```python
from build123d import *

# Parameters (mm, degrees)
SKETCH1_R           = 3.175
BOSS_EXTRUDE1_DEPTH = 6.35


with BuildPart() as part:
    # Sketch1 → Boss-Extrude1 (new body)
    with BuildSketch(Plane.XY):
        Polygon((-63.5, 12.7), (-63.5, 6.35), (-69.85, 6.35), (-69.85, -6.35), (-63.5, -6.35), (-63.5, -12.7), (-57.15, -12.7), (-57.15, -6.35), (-50.8, -6.35), (-50.8, -12.7), (-44.45, -12.7), (-44.45, -6.35), (-38.1, -6.35), (-38.1, -12.7), (-31.75, -12.7), (-31.75, -6.35), (-25.4, -6.35), (-25.4, -12.7), (-19.05, -12.7), (-19.05, -6.35), (-12.7, -6.35), (-12.7, -12.7), (-6.35, -12.7), (-6.35, -6.35), (0, -6.35), (6.35, -6.35), (6.35, -12.7), (12.7, -12.7), (12.7, -6.35), (19.05, -6.35), (19.05, -12.7), (25.4, -12.7), (25.4, -6.35), (31.75, -6.35), (31.75, -12.7), (38.1, -12.7), (38.1, -6.35), (44.45, -6.35), (44.45, -12.7), (50.8, -12.7), (50.8, -6.35), (57.15, -6.35), (57.15, -12.7), (63.5, -12.7), (63.5, -6.35), (69.85, -6.35), (69.85, 6.35), (63.5, 6.35), (63.5, 12.7), (57.15, 12.7), (57.15, 6.35), (50.8, 6.35), (50.8, 12.7), (44.45, 12.7), (44.45, 6.35), (38.1, 6.35), (38.1, 12.7), (31.75, 12.7), (31.75, 6.35), (25.4, 6.35), (25.4, 12.7), (19.05, 12.7), (19.05, 6.35), (12.7, 6.35), (12.7, 12.7), (6.35, 12.7), (6.35, 6.35), (0, 6.35), (-6.35, 6.35), (-6.35, 12.7), (-12.7, 12.7), (-12.7, 6.35), (-19.05, 6.35), (-19.05, 12.7), (-25.4, 12.7), (-25.4, 6.35), (-31.75, 6.35), (-31.75, 12.7), (-38.1, 12.7), (-38.1, 6.35), (-44.45, 6.35), (-44.45, 12.7), (-50.8, 12.7), (-50.8, 6.35), (-57.15, 6.35), (-57.15, 12.7), align=None)
        with Locations((-50.8, 0)):
            Circle(SKETCH1_R, mode=Mode.SUBTRACT)
        with Locations((50.8, 0)):
            Circle(SKETCH1_R, mode=Mode.SUBTRACT)
    extrude(amount=BOSS_EXTRUDE1_DEPTH)


solid = part.part
```
Geometry check sheet. Reference: the model listing, model coordinates, mm. A direction names the side the tool comes from. Round coordinates to 2 decimals unless told otherwise and drop trailing zeros. Order: outer loops, then holes, each group sorted by start corner. A loop starts at its lowest first (then second) coordinate and runs counter-clockwise, first axis right, second up. Notation, with made-up numbers: (-2, 2.5) - (4, 2.5) arc R20 ccw to (4, 15.5) - close; hole circle Ø7 at (-17, 75.25). An arc over 180 degrees is marked (long way). Use a Markdown table: item, result. Add a question column.
(1) Material ranges on line 1 along X through (y, z) = (0.25, 2.25); line 2 along X through (y, z) = (2.25, 3.75); line 3 along Y through (x, z) = (2.5, 4.25), recorded low to high. Write a range as [from, to].
(2) Depth check by flat-ended pin: pin 1 (2 mm diameter, centred on x = 14.5, z = 4, fed in from +Y); pin 2 (8 mm diameter, centred on x = 39, y = -7.5, fed in from -Z); pin 3 (1.9 mm diameter, centred on y = -8.5, z = 3.5, fed in from +X); pin 4 (3 mm diameter, centred on y = 9, z = 4.5, fed in from -X). Enter the tip coordinate at first touch or a pass-through.
(3) Tool access check on faces 1 (the flat face through (41, -6.35, 3)), 2 (the flat face through (-6.35, 9, 3)), 3 (the flat face through (-67, -6.35, 3)). Record the directions out of +Z, -Z, +X, -X, +Y, -Y that give a thin tool (end or side, any length) a straight path to the whole face; none if there is none.
(4) Sectioned sample at B-B, the plane x = -49.5. Enter the section's corners in (y, z), and give its area (3 significant figures).
(5) Sectioned sample at C-C, the plane z = 2. Count the separate pieces of the cut face and the enclosed holes in it, and give its area (3 significant figures).
(6) Sectioned sample at A-A, the plane y = 0. Enter the section's corners in (x, z) (3 decimals).
(7) Release check for a two-part mould opening along X. For faces 4 (the flat face through (57.15, 10, 3)), 5 (the flat face through (69.85, 0, 3)), 6 (the flat face through (48, -12.7, 3)) record: pulls with the +X half, pulls with the -X half, needs draft (parallel to the pull), parting line crosses it, or undercut.
Answers below:
| question | item | result |
|---|---|---|
| 1 | line 1 | [-69.85, -53.97], [-47.63, 47.63], [53.97, 69.85] |
| 1 | line 2 | [-69.85, -53.04], [-48.56, 48.56], [53.04, 69.85] |
| 1 | line 3 | [-6.35, 6.35] |
| 2 | pin 1 | y = 6.35 |
| 2 | pin 2 | z = 0 |
| 2 | pin 3 | x = 63.5 |
| 2 | pin 4 | x = -63.5 |
| 3 | face 1 | +Z, -Z, -Y |
| 3 | face 2 | +Z, -Z, +Y |
| 3 | face 3 | +Z, -Z, -X, -Y |
| 4 | outline | (-12.7, 0) - (-2.9, 0) - (-2.9, 6.35) - (-12.7, 6.35) - close; (2.9, 0) - (12.7, 0) - (12.7, 6.35) - (2.9, 6.35) - close |
| 4 | area | 125 mm² |
| 5 | separate pieces | 1 |
| 5 | enclosed holes | 2 |
| 5 | area | 2,520 mm² |
| 6 | outline | (-69.85, 0) - (-53.975, 0) - (-53.975, 6.35) - (-69.85, 6.35) - close; (-47.625, 0) - (47.625, 0) - (47.625, 6.35) - (-47.625, 6.35) - close; (53.975, 0) - (69.85, 0) - (69.85, 6.35) - (53.975, 6.35) - close |
| 7 | face 4 | undercut |
| 7 | face 5 | pulls with the +X half |
| 7 | face 6 | needs draft |
